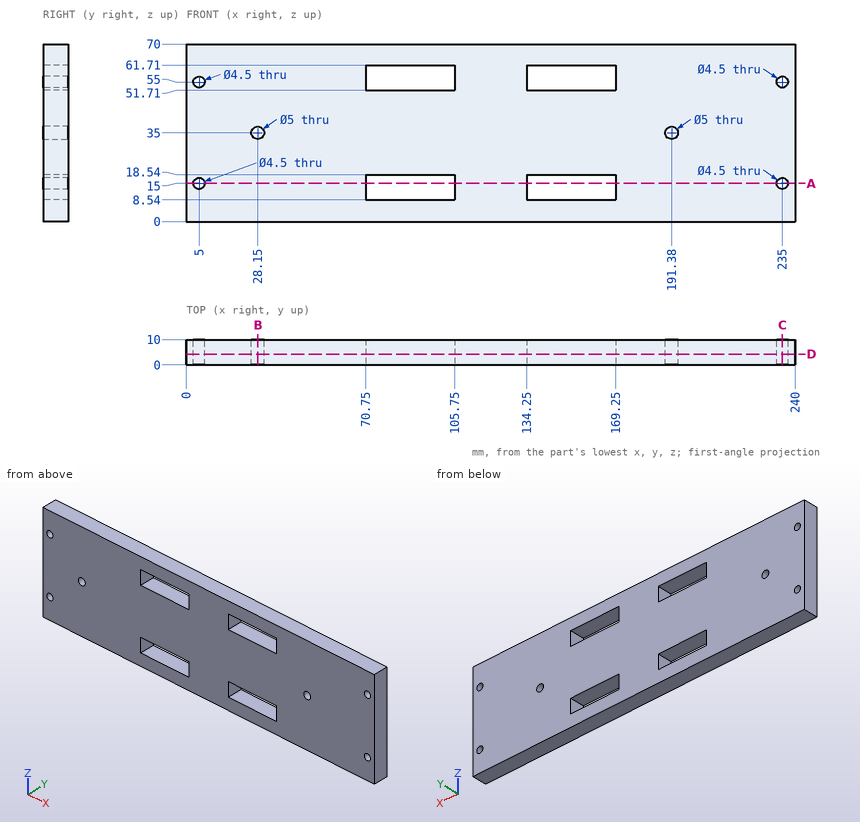
Could you check a few things on this drawing? It's one solid part, dimensions in mm from its lowest x, y, z. Coordinates: 2 decimals unless noted, no trailing zeros. Write each loop counter-clockwise with the first axis right and the second up, starting at its lowest first coordinate (ties: lowest second). Pieces come first, ordered by that corner, then holes.
Q1. Please list where these lines run through material, in increasing order: L1, parallel to Z at x = 5, y = 8; L2, parallel to X at y = 6, z = 15; L3, parallel to Z at x = 167, y = 1.5.
Results found:
L1: z = 0 to 12.75, 17.25 to 52.75, 57.25 to 70
L2: x = 0 to 2.75, 7.25 to 70.75, 105.75 to 134.25, 169.25 to 232.75, 237.25 to 240
L3: z = 0 to 8.54, 18.54 to 51.71, 61.71 to 70
Q2. Imagine slicing it at D-D, the plane y = 4.25. Count the separate pieces of the cut face and the enclosed holes in it, plus the area to 3 significant figures.
Results found:
separate pieces: 1
enclosed holes: 10
area: 15,300 mm2
Q3. Imagine slicing it at B-B, the plane x = 28.15. List the corners of the cut face in (y, z) for me, plus the area to 3 significant figures.
Results found:
outline: (0, 0) - (10, 0) - (10, 32.5) - (0, 32.5) - close; (0, 37.5) - (10, 37.5) - (10, 70) - (0, 70) - close
area: 650 mm2
Q4. Imagine slicing it at A-A, the plane z = 15. List the corners of the cut face in (x, y) for me.
Results found:
outline: (0, 0) - (2.75, 0) - (2.75, 10) - (0, 10) - close; (7.25, 0) - (70.75, 0) - (70.75, 10) - (7.25, 10) - close; (105.75, 0) - (134.25, 0) - (134.25, 10) - (105.75, 10) - close; (169.25, 0) - (232.75, 0) - (232.75, 10) - (169.25, 10) - close; (237.25, 0) - (240, 0) - (240, 10) - (237.25, 10) - close
Q5. Imagine slicing it at C-C, the plane x = 235. List the corners of the cut face in (y, z) for me.
Results found:
outline: (0, 0) - (10, 0) - (10, 12.75) - (0, 12.75) - close; (0, 17.25) - (10, 17.25) - (10, 52.75) - (0, 52.75) - close; (0, 57.25) - (10, 57.25) - (10, 70) - (0, 70) - close
